```python
from build123d import *

# Parameters (mm, degrees)
SKETCH1_W                  = 215
SKETCH1_H                  = 160
BOSS_EXTRUDE1_DEPTH        = 4
F_1_0_3_2_DIAMETER_HOLE1_D = 3.2
FILLET1_R                  = 40
FILLET2_R                  = 40
SKETCH8_R                  = 1.6
CUT_EXTRUDE1_DEPTH         = 135.060620616


with BuildPart() as part:
    # Sketch1 → Boss-Extrude1 (new body)
    with BuildSketch(Plane(origin=(0, 0, 0), x_dir=(1, 0, 0), z_dir=(0, 1, 0))):
        Rectangle(SKETCH1_W, SKETCH1_H)
    extrude(amount=BOSS_EXTRUDE1_DEPTH)

    # Ø1.0 (3.2) Diameter Hole1 (through all)
    with Locations(Plane.XZ):
        with Locations((-70, 55), (33, 55), (-33, 55), (70, 55), (70, -55), (33, -55), (-33, -55), (-70, -55)):
            Hole(F_1_0_3_2_DIAMETER_HOLE1_D / 2)

    # Fillet1
    fillet1_edges = [part.edges().sort_by_distance(p)[0] for p in [
        (-107.5, 2, 80),
        (-107.5, 2, -80),
    ]]
    fillet(fillet1_edges, radius=FILLET1_R)

    # Fillet2
    fillet2_edges = [part.edges().sort_by_distance(p)[0] for p in [
        (107.5, 2, -80),
        (107.5, 2, 80),
    ]]
    fillet(fillet2_edges, radius=FILLET2_R)

    # Sketch8 → Cut-Extrude1 (cut, through all)
    with BuildSketch(Plane.XZ):
        with Locations(Location((-70, -45, 0), (0, 0, 270))):
            Circle(SKETCH8_R)
        with Locations(Location((0, -45, 0), (0, 0, 270))):
            Circle(SKETCH8_R)
        with Locations(Location((70, -45, 0), (0, 0, 270))):
            Circle(SKETCH8_R)
        with Locations(Location((70, 45, 0), (0, 0, 90))):
            Circle(SKETCH8_R)
        with Locations(Location((0, 45, 0), (0, 0, 90))):
            Circle(SKETCH8_R)
        with Locations(Location((-70, 45, 0), (0, 0, 90))):
            Circle(SKETCH8_R)
    extrude(amount=-CUT_EXTRUDE1_DEPTH, mode=Mode.SUBTRACT)


solid = part.part
```
The model under review builds one solid part; all positions refer to its coordinate system, in mm. Coordinates: 2 decimals unless noted, no trailing zeros. Write each loop counter-clockwise with the first axis right and the second up, starting at its lowest first coordinate (ties: lowest second). Pieces come first, ordered by that corner, then holes. Notation, with made-up numbers: (61.5, -24) - (82.5, -24) arc R19 cw to (82.5, -16) - close; hole circle Ø11 at (83.5, 29). An arc over 180 degrees is marked (long way). Answer in a Markdown table with one row per item. Add a question column.
Q1. To check wall thickness, follow line 1 along Z through (x, y) = (33, 1.05); line 2 along X through (y, z) = (1.8, 45); line 3 along Z through (x, y) = (-70, 2.8). State the ranges of each line that lie inside material, in increasing order. Write a range as from..to.
Q2. Consider section B-B on x = -89.5. Give the boundary of the cut face in (y, z), then the cut area to 3 significant figures.
Q3. Consider section A-A on y = 3.15. Give the number of separate pieces and of enclosed holes in the cut face, then the cut area to 3 significant figures.
Answers below:
| question | item | result |
|---|---|---|
| 1 | line 1 | -80..-56.6, -53.4..53.4, 56.6..80 |
| 1 | line 2 | -107.19..-71.6, -68.4..-1.6, 1.6..68.4, 71.6..107.19 |
| 1 | line 3 | -79.92..-56.6, -53.4..-46.6, -43.4..43.4, 46.6..53.4, 56.6..79.92 |
| 2 | outline | (0, -73.41) - (4, -73.41) - (4, 73.41) - (0, 73.41) - close |
| 2 | area | 587 mm² |
| 3 | separate pieces | 1 |
| 3 | enclosed holes | 14 |
| 3 | area | 32,900 mm² |
